Check sheet for the modelled part. Datum: model origin and axes. Units: mm. Face numbers are marked on the shaded views. Round coordinates to 2 decimals unless told otherwise and drop trailing zeros. Write each loop counter-clockwise with the first axis right and the second up, starting at its lowest first coordinate (ties: lowest second). Pieces come first, ordered by that corner, then holes. Notation, with made-up numbers: (-10.5, 36.25) - (26.5, 36.25) arc R12 cw to (26.5, 40.25) - close; hole circle Ø9 at (62, -29). An arc over 180 degrees is marked (long way). Answer as a JSON object with one key per item and string values. Group by question number.
Item 1: Sectioned sample at D-D on y = 2. Record the boundary of the cut face in (x, z).
Item 2: Thickness scan on line 1 (Y direction, x = 23, z = 1.4); line 2 (Y direction, x = 8.5, z = 1.4); line 3 (Y direction, x = 3, z = 1.2). Record the ranges inside material, lowest first.
Item 3: Gauge pin test, flat ends, axial feed: P1, Ø4, axis at x = 2, y = 14.5, coming from the +Z side; P2, Ø2, axis at x = 23, y = 2, coming from the -Z side; P3, Ø0.6, axis at x = 11, z = 1, coming from the -Y side. Record the tip position at first contact, or that the pin passes through.
Item 4: Sectioned sample at B-B on z = 1.55. Record the boundary of the cut face in (x, y).
Item 5: Release check for a two-part mould opening along X. For the marked faces 1, 2 and 3 record: pulls with the +X half, pulls with the -X half, needs draft (parallel to the pull), parting line crosses it, or undercut.
Item 6: Sectioned sample at C-C on y = 14.5. Record the boundary of the cut face in (x, z).
Item 7: Sectioned sample at A-A on x = 11.25. Record the boundary of the cut face in (y, z).
Autodesk Inventor part; units mm, degrees
ref_plane "YZ Plane" through (0, 0, 0) normal (1, 0, 0) x (0, 1, 0)
ref_plane "XZ Plane" through (0, 0, 0) normal (0, 1, 0) x (-1, 0, 0)
ref_plane "XY Plane" through (0, 0, 0) normal (0, 0, 1) x (1, 0, 0)
sketch "Sketch1" plane through (0, 0, 0) normal (0, 0, 1) x (1, 0, 0)
  line L0 (0, 0) -> (25, 0)
  line L1 (25, 0) -> (25, 23.862)
  line L2 (25, 23.862) -> (0, 23.862)
  line L3 (0, 23.862) -> (0, 0)
  circle A0 centre (2, 2) radius 1.25
  circle A1 centre (23, 2) radius 1.25
  circle A2 centre (2, 14.5) radius 1.25
  circle A3 centre (23, 14.5) radius 1.25
  line L4 (7.5, 19.862) -> (17.5, 19.862)
  line L5 (17.5, 19.862) -> (17.5, 9.862)
  line L6 (17.5, 9.862) -> (7.5, 9.862)
  line L7 (7.5, 9.862) -> (7.5, 19.862)
  line L8 (0, 23.862) -> (7.5, 19.862) construction
  line L9 (17.5, 19.862) -> (25, 23.862) construction
  dimension "d0" = 25
  dimension "d1" = 23.862
  dimension "d2" = 2.5
  dimension "d3" = 2
  dimension "d4" = 2
  dimension "d5" = 14.5
  dimension "d6" = 2
  dimension "d7" = 10
  dimension "d8" = 4
extrude "Extrusion1" add sketch "Sketch1" along normal blind 2
fillet "Fillet1" radius 2 4 edges at (25, 23.862, 1) (0, 23.862, 1) (0, 0, 1) (25, 0, 1)
sketch "Sketch2" plane through (0, 0, 2) normal (0, 0, 1) x (1, 0, 0)
  circle A0 centre (2, 14.5) radius 1.25
  circle A1 centre (2, 2) radius 1.25
  circle A2 centre (23, 2) radius 1.25
  circle A3 centre (23, 14.5) radius 1.25
  circle A4 centre (2, 14.5) radius 2.85
  circle A5 centre (2, 2) radius 2.85
  circle A6 centre (23, 2) radius 2.85
  circle A7 centre (23, 14.5) radius 2.85
  point P0 (0, 0)
  dimension "d12" = 1.6
extrude "Extrusion2" add sketch "Sketch2" against normal up to surface (2 mm away)
fillet "Fillet2" radius 2 8 edges at (0, 16.5304, 1) (0, 12.4696, 1) (0, 4.0304, 1) (4.0304, 0, 1) (20.9696, 0, 1) (25, 4.0304, 1) (25, 16.5304, 1) (25, 12.4696, 1)
properties part number "CameraFilterPlate"
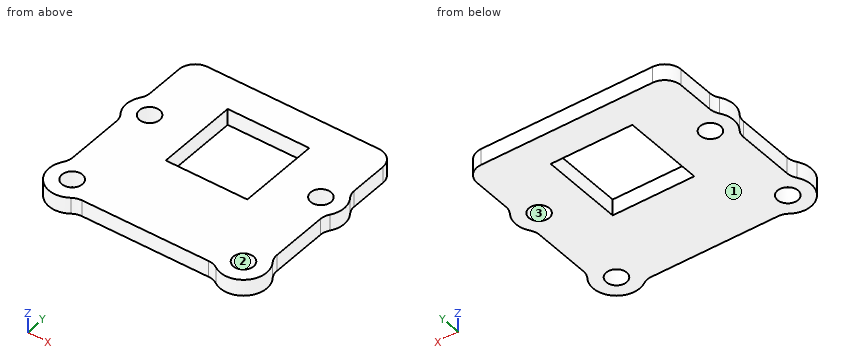
Completed:
{
 "1": {"outline": "(-0.85, 0) - (0.75, 0) - (0.75, 2) - (-0.85, 2) - close; (3.25, 0) - (21.75, 0) - (21.75, 2) - (3.25, 2) - close; (24.25, 0) - (25.85, 0) - (25.85, 2) - (24.25, 2) - close"},
 "2": {"line 1": "-0.85 to 0.75, 3.25 to 13.25, 15.75 to 23.86", "line 2": "0 to 9.86, 19.86 to 23.86", "line 3": "-0.67 to 1.25, 2.75 to 13.75, 15.25 to 23.86"},
 "3": {"P1": "z = 2", "P2": "through", "P3": "y = 0"},
 "4": {"outline": "(-0.35, 3.61) arc R2.85 ccw to (3.61, -0.35) arc R2 cw to (4.74, 0) - (20.26, 0) arc R2 cw to (21.39, -0.35) arc R2.85 ccw to (25.35, 3.61) arc R2 cw to (25, 4.74) - (25, 11.76) arc R2 cw to (25.35, 12.89) arc R2.85 ccw to (25.35, 16.11) arc R2 cw to (25, 17.24) - (25, 21.86) arc R2 ccw to (23, 23.86) - (2, 23.86) arc R2 ccw to (0, 21.86) - (0, 17.24) arc R2 cw to (-0.35, 16.11) arc R2.85 ccw to (-0.35, 12.89) arc R2 cw to (0, 11.76) - (0, 4.74) arc R2 cw to start; hole circle Ø2.5 at (2, 2); hole circle Ø2.5 at (2, 14.5); hole (7.5, 9.86) - (17.5, 9.86) - (17.5, 19.86) - (7.5, 19.86) - close; hole circle Ø2.5 at (23, 2); hole circle Ø2.5 at (23, 14.5)"},
 "5": {"face 1": "needs draft", "face 2": "undercut", "face 3": "undercut"},
 "6": {"outline": "(-0.85, 0) - (0.75, 0) - (0.75, 2) - (-0.85, 2) - close; (3.25, 0) - (7.5, 0) - (7.5, 2) - (3.25, 2) - close; (17.5, 0) - (21.75, 0) - (21.75, 2) - (17.5, 2) - close; (24.25, 0) - (25.85, 0) - (25.85, 2) - (24.25, 2) - close"},
 "7": {"outline": "(0, 0) - (9.86, 0) - (9.86, 2) - (0, 2) - close; (19.86, 0) - (23.86, 0) - (23.86, 2) - (19.86, 2) - close"}
}
